CAD build for the part. Positions are in the model's coordinates, mm. A direction names the side the tool comes from. Coordinates: 2 decimals unless noted, no trailing zeros. Loops run counter-clockwise (first coordinate to the right, second up) from the corner with the lowest first, then second, coordinate; pieces in that order, holes last. Notation, with made-up numbers: (-39, -36.5) -> (2, -36.5) arc R16 ccw to (2, -14.5) -> close; hole circle Ø3 at (-7.75, 45). An arc over 180 degrees is marked (long way). Write each question's results on one line, items separated by ' | '.
from build123d import *

# Parameters (mm, degrees)
SKETCH1_W           = 1.2
SKETCH1_H           = 10
SKETCH1_W_2         = 19
SKETCH1_H_2         = 1.2
BOSS_EXTRUDE1_DEPTH = 349
SKETCH3_R           = 4
CUT_EXTRUDE2_DEPTH  = 370
SKETCH6_W           = 18.962067398
SKETCH6_H           = 10
CUT_EXTRUDE4_DEPTH  = 370
SKETCH10_W          = 1.2
SKETCH10_H          = 10
CUT_EXTRUDE5_DEPTH  = 105


with BuildPart() as part:
    # Sketch1 → Boss-Extrude1 (new body)
    with BuildSketch(Plane.XY):
        Rectangle(SKETCH1_W, SKETCH1_H)
        with Locations((0, -5.6)):
            Rectangle(SKETCH1_W_2, SKETCH1_H_2)
        with Locations((0, 5.6)):
            Rectangle(SKETCH1_W_2, SKETCH1_H_2)
    extrude(amount=BOSS_EXTRUDE1_DEPTH)

    # Sketch3 → Cut-Extrude2 (cut)
    with BuildSketch(Plane(origin=(0, 6.2, 0), x_dir=(1, 0, 0), z_dir=(0, 1, 0))):
        with BuildLine():
            Line((-9.5, 0), (-9.5, -9.5))
            ThreePointArc((-9.5, -9.5), (-6.717514436, -2.782485594), (-4.2e-08, 0))
            Line((-4.2e-08, 0), (-9.5, 0))
        make_face()
        with BuildLine():
            Line((9.5, 0), (-4.2e-08, 0))
            ThreePointArc((-4.2e-08, 0), (6.717514406, -2.782485564), (9.5, -9.5))
            Line((9.5, -9.5), (9.5, 0))
        make_face()
        with BuildLine():
            ThreePointArc((14.5, -9.5), (0, 5), (-14.5, -9.5))
            Line((-14.5, -9.5), (-9.5, -9.5))
            Line((-9.5, -9.5), (-9.5, 0))
            Line((-9.5, 0), (-4.2e-08, 0))
            Line((-4.2e-08, 0), (9.5, 0))
            Line((9.5, 0), (9.5, -9.5))
            Line((9.5, -9.5), (14.5, -9.5))
        make_face()
        with Locations((0, -9.5)):
            Circle(SKETCH3_R)
    cut_extrude2 = extrude(amount=-CUT_EXTRUDE2_DEPTH, mode=Mode.SUBTRACT)

    # Mirror1: Cut-Extrude2 across plane
    add(cut_extrude2.mirror(Plane.XY.offset(174.5)), mode=Mode.SUBTRACT)

    # Sketch6 → Cut-Extrude4 (cut)
    with BuildSketch(Plane.ZY.offset(0.6)):
        with Locations((9.5, 0)):
            Rectangle(SKETCH6_W, SKETCH6_H)
    extrude(amount=-CUT_EXTRUDE4_DEPTH, mode=Mode.SUBTRACT)

    # Sketch10 → Cut-Extrude5 (cut)
    with BuildSketch(Plane(origin=(0, 0, 18.981033699), x_dir=(-1, 0, 0), z_dir=(0, 0, -1))):
        Rectangle(SKETCH10_W, SKETCH10_H)
    cut_extrude5 = extrude(amount=CUT_EXTRUDE5_DEPTH, mode=Mode.SUBTRACT)

    # Mirror2: Cut-Extrude5 across plane
    add(cut_extrude5.mirror(Plane.XY.offset(174.5)), mode=Mode.SUBTRACT)


solid = part.part
1) Which spindle directions (+Z, -Z, +X, -X, +Y, -Y) get a long thin tool onto all of the face, cutting with end or side? Do faces 1 (the cylindrical face through (-0.867, -5.592, 13.405)), 2 (the flat face through (-0.6, 0, 172)). Say none if no direction does.
Outcome:
face 1: +Y, -Y | face 2: +Z, -Z, -X
2) Slice it at B-B (y = -2.25). Write the cut outline in (x, z).
Outcome:
outline: (-0.6, 18.98) -> (0.6, 18.98) -> (0.6, 330.02) -> (-0.6, 330.02) -> close
3) Two-plate mould, pull along X, no slides. Class faces 3 (the cylindrical face through (-0.867, 5.608, 13.405)), 4 (the flat face through (-2, -5, 172)), 5 (the flat face through (0.6, 0, 172)): pulls with the +X half, pulls with the -X half, needs draft (parallel to the pull), parting line crosses it, or undercut.
Outcome:
face 3: undercut | face 4: needs draft | face 5: pulls with the +X half
4) Slice it at A-A (z = 146). Write the cut outline in (x, y), then the cut area to 3 significant figures.
Outcome:
outline: (-9.5, -6.2) -> (9.5, -6.2) -> (9.5, -5) -> (0.6, -5) -> (0.6, 5) -> (9.5, 5) -> (9.5, 6.2) -> (-9.5, 6.2) -> (-9.5, 5) -> (-0.6, 5) -> (-0.6, -5) -> (-9.5, -5) -> close | area: 57.6 mm^2
5) Drill centre lines: L1, parallel to Z at x = 0, y = -5.65; L2, parallel to Y at x = 1.5, z = 55.5; L3, parallel to X at y = 5.35, z = 339.5. Where is each one in solid material? Low to high. Write a range as from..to.
Outcome:
L1: z = 0..5.5, 13.5..335.5, 343.5..349 | L2: y = -6.2..-5, 5..6.2 | L3: x = -9.5..-4, 4..9.5
6) Pin check, flat tips, straight feed: pin 1 (1 mm diameter, centred on x = 0, y = 1, fed in from -Z); pin 2 (2 mm diameter, centred on x = -6, y = 4.5, fed in from -Z); pin 3 (3 mm diameter, centred on y = 1, z = 227, fed in from +X). Stop position of each tip, or through.
Outcome:
pin 1: stops at z = 18.98 | pin 2: stops at z = 1.51 | pin 3: stops at x = 0.6
